from build123d import *

# Parameters (mm, degrees)
SKETCH1_R           = 72
BOSS_EXTRUDE1_DEPTH = 600
SKETCH2_W           = 300
SKETCH2_H           = 300
BOSS_EXTRUDE2_DEPTH = 50
SKETCH3_R           = 70
SKETCH3_R_2         = 65
BOSS_EXTRUDE3_DEPTH = 50


with BuildPart() as part:
    # Sketch1 → Boss-Extrude1 (new body)
    with BuildSketch(Plane(origin=(0, 0, 0), x_dir=(1, 0, 0), z_dir=(0, 1, 0))):
        Circle(SKETCH1_R)
    extrude(amount=BOSS_EXTRUDE1_DEPTH)

    # Sketch2 → Boss-Extrude2 (add)
    with BuildSketch(Plane(origin=(0, 600, 0), x_dir=(1, 0, 0), z_dir=(0, 1, 0))):
        Rectangle(SKETCH2_W, SKETCH2_H)
    extrude(amount=BOSS_EXTRUDE2_DEPTH)

    # Sketch3 → Boss-Extrude3 (add)
    with BuildSketch(Plane(origin=(0, 650, 0), x_dir=(1, 0, 0), z_dir=(0, 1, 0))):
        Circle(SKETCH3_R)
        Circle(SKETCH3_R_2, mode=Mode.SUBTRACT)
    extrude(amount=BOSS_EXTRUDE3_DEPTH)


solid = part.part
Source: CAD feature listing. Evaluate the final solid. Frame: model axes, mm. A direction names the side the tool comes from. Round coordinates to 2 decimals unless told otherwise and drop trailing zeros. Loops run counter-clockwise (first coordinate to the right, second up) from the corner with the lowest first, then second, coordinate; pieces in that order, holes last. Notation, with made-up numbers: M 35.5,-12.75 L 62.5,-12.75 A28 ccw 62.5,13.25 Z; hole C -38.75,1.25 d11. An arc over 180 degrees is marked long. Return JSON: item names as keys, results as strings. Group by question number.
1. Section query B-B on x = 0. Output: boundary loops of the cut face in (y, z).
2. Mould query, pull axis X, two halves, no side actions, for faces 1 (the face through (-1, 650, -1)), 2 (the face through (-150, 625, 2)), 3 (the face through (-2, 625, -150)). Classes: released by +X, released by -X, zero draft, split by the parting line, or undercut.
3. Material intervals for line 1 along Z through (x, y) = (0, 682); line 2 along Y through (x, z) = (26, -3.5), sorted ascending. Write a range as from..to.
4. Pin query (flat end, axial travel): pin 1 (12 mm diameter, centred on x = -83, z = 94.5, fed in from +Y); pin 2 (2 mm diameter, centred on y = 486.5, z = -60, fed in from -X); pin 3 (1.5 mm diameter, centred on y = 167, z = 25, fed in from +X). Return the tip coordinate at first contact, or that it passes through.
5. Section query C-C on y = 248. Output: boundary loops of the cut face in (x, z), and give its area (3 significant figures).
6. Section query D-D on x = 101.5. Output: boundary loops of the cut face in (y, z), and give its area (3 significant figures).
7. Section query A-A on z = 0. Output: boundary loops of the cut face in (x, y), and give its area (3 significant figures).
8. Reachability of faces 4 (the face through (-9.373, 295.8, -71.387)), 5 (the face through (-35, 650, 65)), 6 (the face through (20.4, 700, 61.9)) from +Z, -Z, +X, -X, +Y, -Y: full face, straight path, thin tool, end or side. Return the list, or none.
Checks:
{
 "1": {"outline": "M 0,-72 L 600,-72 L 600,-150 L 650,-150 L 650,-70 L 700,-70 L 700,-65 L 650,-65 L 650,65 L 700,65 L 700,70 L 650,70 L 650,150 L 600,150 L 600,72 L 0,72 Z"},
 "2": {"face 1": "undercut", "face 2": "released by -X", "face 3": "zero draft"},
 "3": {"line 1": "z = -70..-65, 65..70", "line 2": "y = 0..650"},
 "4": {"pin 1": "stops at y = 650", "pin 2": "stops at x = -41.27", "pin 3": "stops at x = 67.79"},
 "5": {"outline": "C 0,0 d144", "area": "16,300 mm²"},
 "6": {"outline": "M 600,-150 L 650,-150 L 650,150 L 600,150 Z", "area": "15,000 mm²"},
 "7": {"outline": "M -150,600 L -72,600 L -72,0 L 72,0 L 72,600 L 150,600 L 150,650 L 70,650 L 70,700 L 65,700 L 65,650 L -65,650 L -65,700 L -70,700 L -70,650 L -150,650 Z", "area": "102,000 mm²"},
 "8": {"face 4": "-Y", "face 5": "+Y", "face 6": "+Z, -Z, +X, -X, +Y"}
}
